from build123d import *

# Parameters (mm, degrees)
SKETCH1_W               = 18
SKETCH1_H               = 5
BOSS_EXTRUDE1_DEPTH     = 15
SKETCH2_R               = 1.5
CUT_EXTRUDE1_DEPTH      = 20
SKETCH3_R               = 1.5
CUT_EXTRUDE2_DEPTH      = 15
CUT_EXTRUDE3_DEPTH      = 290
CUT_EXTRUDE3_DEPTH_BACK = 330
SKETCH4_R               = 4.05
LPATTERN3_COUNT         = 6
LPATTERN3_PITCH         = 12.25
LPATTERN4_COUNT         = 6
LPATTERN4_PITCH         = 12.25
FILLET1_R               = 5
FILLET2_R               = 5
FILLET3_R               = 5
FILLET4_R               = 5
FILLET5_R               = 1.5
FILLET6_R               = 1.5


# Some blends are built 0.0001 mm under size
with BuildPart() as part:
    # Sketch1 → Boss-Extrude1 (new body)
    with BuildSketch(Plane.XY):
        with BuildLine():
            ThreePointArc((94.967099566, 2.5), (0, 95), (-94.967099566, 2.5))
            Line((-94.967099566, 2.5), (-89.965271077, 2.5))
            ThreePointArc((-89.965271077, 2.5), (0, 90), (89.965271077, 2.5))
            Line((89.965271077, 2.5), (94.967099566, 2.5))
        make_face()
        with BuildLine():
            Line((-89.965271077, -2.5), (-94.967099566, -2.5))
            ThreePointArc((-94.967099566, -2.5), (0, -95), (94.967099566, -2.5))
            Line((94.967099566, -2.5), (89.965271077, -2.5))
            ThreePointArc((89.965271077, -2.5), (0, -90), (-89.965271077, -2.5))
        make_face()
        with BuildLine():
            Line((-94.967099566, 2.5), (-94.967099566, -2.5))
            Line((-94.967099566, -2.5), (-89.965271077, -2.5))
            ThreePointArc((-89.965271077, -2.5), (-90, 0), (-89.965271077, 2.5))
            Line((-89.965271077, 2.5), (-94.967099566, 2.5))
        make_face()
        with BuildLine():
            ThreePointArc((-89.965271077, 2.5), (-90, 0), (-89.965271077, -2.5))
            Line((-89.965271077, -2.5), (-9, -2.5))
            Line((-9, -2.5), (-9, 2.5))
            Line((-9, 2.5), (-89.965271077, 2.5))
        make_face()
        with BuildLine():
            Line((9, -2.5), (89.965271077, -2.5))
            ThreePointArc((89.965271077, -2.5), (89.99131735, -1.250120604), (90, 0))
            ThreePointArc((90, 0), (89.99131735, 1.250120604), (89.965271077, 2.5))
            Line((89.965271077, 2.5), (9, 2.5))
            Line((9, 2.5), (9, -2.5))
        make_face()
        with BuildLine():
            Line((89.965271077, -2.5), (94.967099566, -2.5))
            Line((94.967099566, -2.5), (94.967099566, 2.5))
            Line((94.967099566, 2.5), (89.965271077, 2.5))
            ThreePointArc((89.965271077, 2.5), (89.99131735, 1.250120604), (90, 0))
            ThreePointArc((90, 0), (89.99131735, -1.250120604), (89.965271077, -2.5))
        make_face()
        Rectangle(SKETCH1_W, SKETCH1_H)
        with Locations((0, 5)):
            Rectangle(SKETCH1_W, SKETCH1_H)
        with Locations((0, -5)):
            Rectangle(SKETCH1_W, SKETCH1_H)
    extrude(amount=BOSS_EXTRUDE1_DEPTH)

    # Sketch2 → Cut-Extrude1 (cut)
    with BuildSketch(Plane(origin=(0, 2.5, 0), x_dir=(1, 0, 0), z_dir=(0, 1, 0))):
        with Locations(Location((-82.965271077, -7.5, 0), (0, 0, 270))):
            Circle(SKETCH2_R)
    cut_extrude1 = extrude(amount=-CUT_EXTRUDE1_DEPTH, mode=Mode.SUBTRACT)

    # Sketch3 → Cut-Extrude2 (cut)
    with BuildSketch(Plane(origin=(0, 2.5, 0), x_dir=(1, 0, 0), z_dir=(0, 1, 0))):
        with Locations(Location((82.965271077, -7.5, 0), (0, 0, 270))):
            Circle(SKETCH3_R)
    cut_extrude2 = extrude(amount=-CUT_EXTRUDE2_DEPTH, mode=Mode.SUBTRACT)

    # Sketch4 → Cut-Extrude3 (cut, two sides: drawn at the far end of the back side and taken through both)
    with BuildSketch(Plane(origin=(0, 7.5, 0), x_dir=(1, 0, 0), z_dir=(0, 1, 0)).offset(-CUT_EXTRUDE3_DEPTH_BACK)):
        with Locations(Location((0, -7.5, 0), (0, 0, 90))):
            Circle(SKETCH4_R)
    extrude(amount=CUT_EXTRUDE3_DEPTH + CUT_EXTRUDE3_DEPTH_BACK, mode=Mode.SUBTRACT)

    # LPattern3: Cut-Extrude2 ×6
    with Locations(*[(-i * LPATTERN3_PITCH, 0, 0) for i in range(1, LPATTERN3_COUNT)]):
        add(cut_extrude2, mode=Mode.SUBTRACT)

    # LPattern4: Cut-Extrude1 ×6
    with Locations(*[(i * LPATTERN4_PITCH, 0, 0) for i in range(1, LPATTERN4_COUNT)]):
        add(cut_extrude1, mode=Mode.SUBTRACT)

    # Fillet1
    fillet1_edges = [part.edges().sort_by_distance(p)[0] for p in [
        (-9, 7.5, 7.5),
    ]]
    fillet(fillet1_edges, radius=FILLET1_R - 0.0001)  # a hair under: the kernel refuses the full size

    # Fillet2
    fillet2_edges = [part.edges().sort_by_distance(p)[0] for p in [
        (9, 7.5, 7.5),
    ]]
    fillet(fillet2_edges, radius=FILLET2_R - 0.0001)  # a hair under: the kernel refuses the full size

    # Fillet3
    fillet3_edges = [part.edges().sort_by_distance(p)[0] for p in [
        (9, -7.5, 7.5),
    ]]
    fillet(fillet3_edges, radius=FILLET3_R - 0.0001)  # a hair under: the kernel refuses the full size

    # Fillet4
    fillet4_edges = [part.edges().sort_by_distance(p)[0] for p in [
        (-9, -7.5, 7.5),
    ]]
    fillet(fillet4_edges, radius=FILLET4_R - 0.0001)  # a hair under: the kernel refuses the full size

    # Fillet5
    # the kernel refuses this fillet: 1.5 mm, written as the material it takes off along each edge
    with BuildSketch(Plane(origin=(0, 0, 15), x_dir=(-0.9999126669586381, 0.013215841088011512, 0), z_dir=(0.013215841088011512, 0.9999126669586381, 0))) as fillet5_piece_1:
        with BuildLine():
            CenterArc((95 - FILLET5_R, -FILLET5_R), FILLET5_R, 0, 90)
            Line((95 - FILLET5_R, 0), (95, 0))
            Line((95, 0), (95, -FILLET5_R))
        make_face()
    revolve(axis=Axis((0, 0, 15), (0, 0, 1)), revolution_arc=181.514467922, mode=Mode.SUBTRACT)
    with BuildSketch(Plane(origin=(0, 0, 15), x_dir=(0.9999126669586381, -0.013215841088011463, 0), z_dir=(-0.013215841088011463, -0.9999126669586381, 0))) as fillet5_piece_2:
        with BuildLine():
            CenterArc((95 - FILLET5_R, -FILLET5_R), FILLET5_R, 0, 90)
            Line((95 - FILLET5_R, 0), (95, 0))
            Line((95, 0), (95, -FILLET5_R))
        make_face()
    revolve(axis=Axis((0, 0, 15), (0, 0, 1)), revolution_arc=181.514467922, mode=Mode.SUBTRACT)

    # Fillet6
    # the kernel refuses this fillet: 1.5 mm, written as the material it takes off along each edge
    with BuildSketch(Plane(origin=(0, 0, 0), x_dir=(0.9999126669586381, -0.013215841088011463, 0), z_dir=(-0.013215841088011463, -0.9999126669586381, 0))) as fillet6_piece_1_section:
        with BuildLine():
            CenterArc((95 - FILLET6_R, FILLET6_R), FILLET6_R, 270, 90)
            Line((95, FILLET6_R), (95 + FILLET6_R * 0.02, FILLET6_R))
            Line((95 + FILLET6_R * 0.02, FILLET6_R), (95 + FILLET6_R * 0.02, -FILLET6_R * 0.02))
            Line((95 + FILLET6_R * 0.02, -FILLET6_R * 0.02), (95 - FILLET6_R, -FILLET6_R * 0.02))
            Line((95 - FILLET6_R, -FILLET6_R * 0.02), (95 - FILLET6_R, 0))
        make_face()
    fillet6_piece_1 = revolve(axis=Axis((0, 0, 0), (0, 0, 1)), revolution_arc=181.514467922, mode=Mode.PRIVATE)
    fillet6_piece_1 = split(fillet6_piece_1, bisect_by=Plane(origin=(-94.967099566, 94.599989904, 0.400010096), z_dir=(1, 0, 0)), keep=Keep.TOP, mode=Mode.PRIVATE)
    fillet6_piece_1 = split(fillet6_piece_1, bisect_by=Plane(origin=(94.967099566, 94.599989904, 0.400010096), z_dir=(-1, 0, 0)), keep=Keep.TOP, mode=Mode.PRIVATE)
    with BuildSketch(Plane(origin=(0, 0, 0), x_dir=(-0.9999126669586381, 0.013215841088011512, 0), z_dir=(0.013215841088011512, 0.9999126669586381, 0))) as fillet6_piece_2_section:
        with BuildLine():
            CenterArc((95 - FILLET6_R, FILLET6_R), FILLET6_R, 270, 90)
            Line((95, FILLET6_R), (95 + FILLET6_R * 0.02, FILLET6_R))
            Line((95 + FILLET6_R * 0.02, FILLET6_R), (95 + FILLET6_R * 0.02, -FILLET6_R * 0.02))
            Line((95 + FILLET6_R * 0.02, -FILLET6_R * 0.02), (95 - FILLET6_R, -FILLET6_R * 0.02))
            Line((95 - FILLET6_R, -FILLET6_R * 0.02), (95 - FILLET6_R, 0))
        make_face()
    fillet6_piece_2 = revolve(axis=Axis((0, 0, 0), (0, 0, 1)), revolution_arc=181.514467922, mode=Mode.PRIVATE)
    fillet6_piece_2 = split(fillet6_piece_2, bisect_by=Plane(origin=(-94.967099566, -94.599989904, 0.400010096), z_dir=(1, 0, 0)), keep=Keep.TOP, mode=Mode.PRIVATE)
    fillet6_piece_2 = split(fillet6_piece_2, bisect_by=Plane(origin=(94.967099566, -94.599989904, 0.400010096), z_dir=(-1, 0, 0)), keep=Keep.TOP, mode=Mode.PRIVATE)
    add([fillet6_piece_1, fillet6_piece_2], mode=Mode.SUBTRACT)


solid = part.part
Can you work these out from the model? Positions are in its coordinate system, mm. A direction names the side the tool comes from. Coordinates: 2 decimals unless noted, no trailing zeros. Answer as a JSON object with one key per item and string values. Group by question number.
Item 1: If we mould it in two halves opening along X, with no side actions, what happens to faces 1 (the face through (-2.054, -94.978, 11.416)), 2 (the face through (-1.94, 89.98, 12.4)), 3 (the face through (94.967, 0, 7)), 4 (the face through (0, 7, 15))? For each: released by +X, released by -X, zero draft, split by the parting line, or undercut.
Item 2: For pin 1 (5 mm diameter, centred on x = -70.72, z = 7.5, fed in from -Y); pin 2 (6 mm diameter, centred on y = -74.5, z = 2.5, fed in from +X); pin 3 (2.5 mm diameter, centred on x = -82.97, z = 7.5, fed in from -Y), each with a flat end and sliding along its axis, tell me the tip position at first contact or that it passes through.
Item 3: If I drill on L1, parallel to Y at x = 59.5, z = 11; L2, parallel to Y at x = -19, z = 8.25; L3, parallel to X at y = -26, z = 11, over which ranges is the centre line in solid material (lowest first)? Write a range as from..to.
Item 4: On a 3-axis mill with a long thin cutter (end or side, diameter ignored), from which of +Z, -Z, +X, -X, +Y, -Y can I reach the whole of each face in a straight line? I mean faces 5 (the face through (2.054, 94.978, 11.416)), 6 (the face through (-7.5, -6.07, 11.61)). Say none if no direction works.
Returned:
{
 "1": {"face 1": "split by the parting line", "face 2": "undercut", "face 3": "released by +X", "face 4": "zero draft"},
 "2": {"pin 1": "stops at y = -66.11", "pin 2": "stops at x = 62.55", "pin 3": "stops at y = -48.44"},
 "3": {"L1": "y = -74.06..-67.53, -2.5..2.5, 67.53..74.06", "L2": "y = -93.08..-87.97, -2.5..2.5, 87.97..93.08", "L3": "x = -91.37..-86.16, 86.16..91.37"},
 "4": {"face 5": "+Z, -Z, +Y", "face 6": "+Z, -Z"}
}
